Could you check a few things on this model? Use its own coordinates, in mm. A direction names the side the tool comes from. Round coordinates to 2 decimals unless told otherwise and drop trailing zeros. Order: outer loops, then holes, each group sorted by start corner. A loop starts at its lowest first (then second) coordinate and runs counter-clockwise, first axis right, second up. Notation, with made-up numbers: M 20,48.25 L 48,48.25 A24 ccw 48,68.25 Z; hole C 54,37.25 d7. An arc over 180 degrees is marked long. Write each question's results on one line, items separated by ' | '. Start each with the question number.
1. Please list where these lines run through material, in increasing order: L1, parallel to X at y = 10.25, z = -32.5; L2, parallel to Z at x = 20.5, y = 2.75 (3 decimals); L3, parallel to Y at x = 59, z = -50.5.
2. We'd pull the mould along Z, two halves only. Please class faces 1 (the flat face through (46, 1.588, -4)), 2 (the flat face through (47, 6, -60.325)), 3 (the flat face through (46, 0, -35)): released by +Z, released by -Z, zero draft, split by the parting line, or undercut.
3. Suppose I cut it at D-D on y = 8.25. Write out the boundary of the cut face in (x, z) (3 decimals), and give its area (3 significant figures).
4. I'm going to push flat-ended pins straight in: pin 1 (1.2 mm diameter, centred on y = 3, z = -1, fed in from +X); pin 2 (3 mm diameter, centred on y = 7.5, z = -25.5, fed in from -X); pin 3 (6 mm diameter, centred on y = 6, z = -19.5, fed in from +X). Where does each tip first touch, or does it pass through?
5. For faces 4 (the flat face through (86.519, 6, -35)), 5 (the flat face through (12.7, 3, -1)), 6 (the flat face through (63.5, 3, -1)), 7 (the flat face through (38, 3.969, -1)), which set-ups out of +Z, -Z, +X, -X, +Y, -Y let a thin tool reach every point of the face, with its end or its side?
6. Suppose I cut it at C-C on z = -42.5. Write out the boundary of the cut face in (x, y).
7. Suppose I cut it at A-A on z = -11. Write out the boundary of the cut face in (x, y), and give its area (3 significant figures).
from build123d import *

# Parameters (mm, degrees)
SKETCH1_W           = 93.6625
SKETCH1_H           = 69.85
SKETCH1_R           = 1.5875
BOSS_EXTRUDE1_DEPTH = 1.5875
SKETCH2_W           = 77.7875
SKETCH2_H           = 50.8
BOSS_EXTRUDE2_DEPTH = 8.73125
SKETCH3_W           = 50.8
SKETCH3_H           = 2.38125
BOSS_EXTRUDE3_DEPTH = 2.38125
SKETCH4_W           = 71.4375
SKETCH4_H           = 44.45
CUT_EXTRUDE1_DEPTH  = 0.396875


with BuildPart() as part:
    # Sketch1 → Boss-Extrude1 (new body)
    with BuildSketch(Plane(origin=(0, 0, 0), x_dir=(1, 0, 0), z_dir=(0, 1, 0))):
        with Locations((46.83125, 34.925)):
            Rectangle(SKETCH1_W, SKETCH1_H)
        with Locations((2.778125, 67.071875)):
            Circle(SKETCH1_R, mode=Mode.SUBTRACT)
        with Locations((90.884375, 67.071875)):
            Circle(SKETCH1_R, mode=Mode.SUBTRACT)
        with Locations((2.778125, 2.778125)):
            Circle(SKETCH1_R, mode=Mode.SUBTRACT)
        with Locations((90.884375, 2.778125)):
            Circle(SKETCH1_R, mode=Mode.SUBTRACT)
    extrude(amount=BOSS_EXTRUDE1_DEPTH)

    # Sketch2 → Boss-Extrude2 (add)
    with BuildSketch(Plane(origin=(0, 1.5875, 0), x_dir=(1, 0, 0), z_dir=(0, 1, 0))):
        with Locations((47.625, 34.925)):
            Rectangle(SKETCH2_W, SKETCH2_H)
    extrude(amount=BOSS_EXTRUDE2_DEPTH)

    # Sketch3 → Boss-Extrude3 (add)
    with BuildSketch(Plane(origin=(0, 1.5875, 0), x_dir=(1, 0, 0), z_dir=(0, 1, 0))):
        with Locations((38.1, 1.190625)):
            Rectangle(SKETCH3_W, SKETCH3_H)
    extrude(amount=BOSS_EXTRUDE3_DEPTH)

    # Sketch4 → Cut-Extrude1 (cut)
    with BuildSketch(Plane(origin=(0, 10.31875, 0), x_dir=(1, 0, 0), z_dir=(0, 1, 0))):
        with Locations((47.625, 34.925)):
            Rectangle(SKETCH4_W, SKETCH4_H)
    extrude(amount=-CUT_EXTRUDE1_DEPTH, mode=Mode.SUBTRACT)


solid = part.part
Filled sheet:
1) L1: x = 8.73 to 11.91, 83.34 to 86.52 | L2: z = -60.325 to -9.525, -2.381 to 0 | L3: y = 0 to 9.92
2) face 1: undercut | face 2: released by -Z | face 3: zero draft
3) outline: M 8.731,-60.325 L 86.519,-60.325 L 86.519,-9.525 L 8.731,-9.525 Z | area: 3,950 mm^2
4) pin 1: stops at x = 63.5 | pin 2: stops at x = 8.73 | pin 3: stops at x = 86.52
5) face 4: +Z, -Z, +X, +Y | face 5: +Z, -X, +Y | face 6: +Z, +X, +Y | face 7: +Z, +X, -X, +Y
6) outline: M 0,0 L 93.66,0 L 93.66,1.59 L 86.52,1.59 L 86.52,10.32 L 83.34,10.32 L 83.34,9.92 L 11.91,9.92 L 11.91,10.32 L 8.73,10.32 L 8.73,1.59 L 0,1.59 Z
7) outline: M 0,0 L 93.66,0 L 93.66,1.59 L 86.52,1.59 L 86.52,10.32 L 8.73,10.32 L 8.73,1.59 L 0,1.59 Z | area: 828 mm^2
